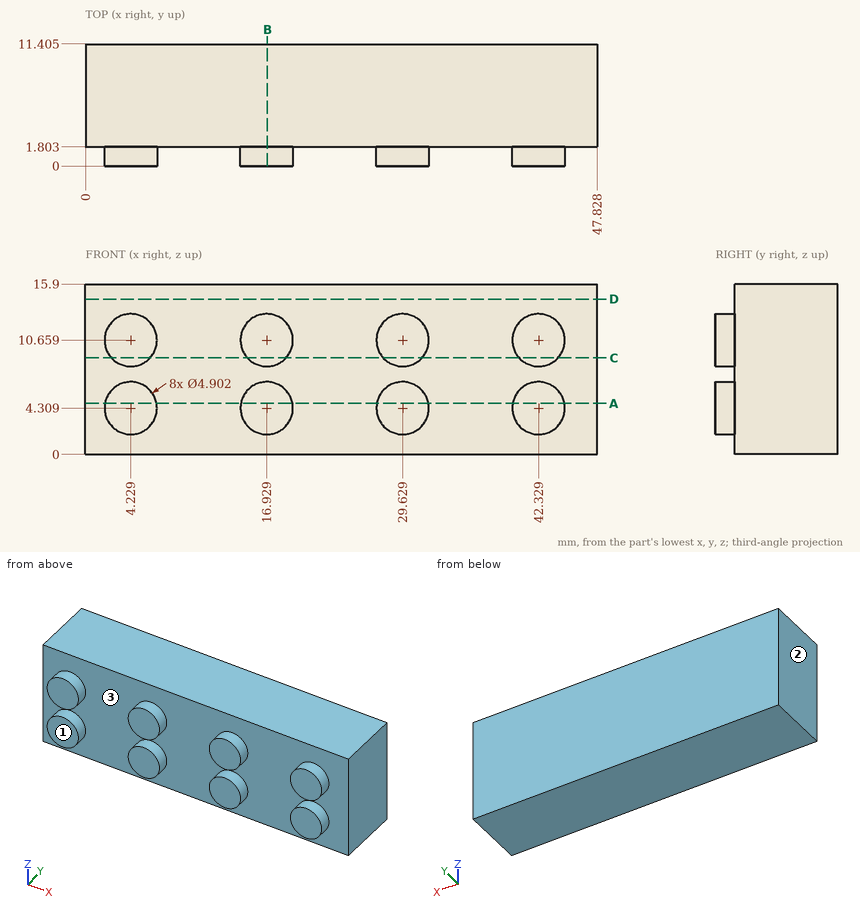
Design review of the part shown in the three views and the two pictorial views. Dimensions are in mm from the part's minimum x, y and z. Round coordinates to 2 decimals unless told otherwise and drop trailing zeros. Loops run counter-clockwise (first coordinate to the right, second up) from the corner with the lowest first, then second, coordinate; pieces in that order, holes last. Notation, with made-up numbers: (27, 78.25) -> (65, 78.25) arc R15 cw to (65, 83.25) -> close; hole circle Ø2 at (-9, 46.25). An arc over 180 degrees is marked (long way). Answer as a JSON object with one key per item and string values. Group by question number.
1) We need section D-D on z = 14.5. Write out the cut boundary in (x, y) (1 decimal).
2) We need section C-C on z = 9. Write out the cut boundary in (x, y) (1 decimal), then the cut area to 3 significant figures.
3) For line 1 (X direction, y = 1, z = 12.25) (1 decimal); line 2 (Y direction, x = 36.5, z = 7.5) (1 decimal), list the stretches that pass through material, from the lowest coordinate up. Write a range as [from, to].
4) We need section B-B on x = 17. Write out the cut boundary in (y, z) (1 decimal).
5) We need section A-A on z = 4.75. Write out the cut boundary in (x, y) (1 decimal), then the cut area to 3 significant figures.
6) Mouldability with a two-part tool opening along X and no side actions: class the marked faces 1, 2 and 3 as released by +X, released by -X, zero draft, split by the parting line, or undercut.
Result set:
{
 "1": {"outline": "(0, 1.8) -> (47.8, 1.8) -> (47.8, 11.4) -> (0, 11.4) -> close"},
 "2": {"outline": "(0, 1.8) -> (2.4, 1.8) -> (2.4, 0) -> (6, 0) -> (6, 1.8) -> (15.1, 1.8) -> (15.1, 0) -> (18.7, 0) -> (18.7, 1.8) -> (27.8, 1.8) -> (27.8, 0) -> (31.4, 0) -> (31.4, 1.8) -> (40.5, 1.8) -> (40.5, 0) -> (44.1, 0) -> (44.1, 1.8) -> (47.8, 1.8) -> (47.8, 11.4) -> (0, 11.4) -> close", "area": "485 mm²"},
 "3": {"line 1": "[2.4, 6.1], [15.1, 18.8], [27.8, 31.5], [40.5, 44.2]", "line 2": "[1.8, 11.4]"},
 "4": {"outline": "(0, 1.9) -> (1.8, 1.9) -> (1.8, 0) -> (11.4, 0) -> (11.4, 15.9) -> (1.8, 15.9) -> (1.8, 13.1) -> (0, 13.1) -> (0, 8.2) -> (1.8, 8.2) -> (1.8, 6.8) -> (0, 6.8) -> close"},
 "5": {"outline": "(0, 1.8) -> (1.8, 1.8) -> (1.8, 0) -> (6.6, 0) -> (6.6, 1.8) -> (14.5, 1.8) -> (14.5, 0) -> (19.3, 0) -> (19.3, 1.8) -> (27.2, 1.8) -> (27.2, 0) -> (32, 0) -> (32, 1.8) -> (39.9, 1.8) -> (39.9, 0) -> (44.7, 0) -> (44.7, 1.8) -> (47.8, 1.8) -> (47.8, 11.4) -> (0, 11.4) -> close", "area": "494 mm²"},
 "6": {"face 1": "zero draft", "face 2": "released by -X", "face 3": "undercut"}
}
